Verification items for the finished model (mm, model axes). A direction names the side the tool comes from. Give positions to 0.01 mm unless a question says otherwise; leave off trailing zeros. Order: outer loops, then holes, each group sorted by start corner. A loop starts at its lowest first (then second) coordinate and runs counter-clockwise, first axis right, second up.
(1) Gauge pin test, flat ends, axial feed: pin 1 (12 mm diameter, centred on x = -10, z = 9.5, fed in from -Y); pin 2 (1.5 mm diameter, centred on x = 5, z = -1, fed in from -Y); pin 3 (5 mm diameter, centred on x = -10, z = -4, fed in from +Y); pin 4 (1.5 mm diameter, centred on y = 16, z = 3, fed in from +X). Record the tip position at first contact, or that the pin passes through.
(2) Access from +Z, -Z, +X, -X, +Y, -Y to the whole of each face (thin tool, end or side, straight path). Record for faces 1 (the face through (16, 0, 7)), 2 (the face through (-3, 25, 0)), 3 (the face through (0.867, 4.93, 3.905)).
(3) Scan lines: L1, parallel to Z at x = 0, y = 6.25; L2, parallel to X at y = 24.75, z = 0. Record each from-to range of solid material in increasing order.
(4) Sectioned sample at A-A on y = 5. Record the cut outline in (x, z), plus the area to 3 significant figures.
(5) Sectioned sample at D-D on y = 25. Record the cut outline in (x, z), plus the area to 3 significant figures.
(6) Sectioned sample at C-C on x = 0. Record the cut outline in (y, z).
(7) Sectioned sample at B-B on z = 0. Record the cut outline in (x, y).
Autodesk Inventor part; units mm, degrees
ref_plane "YZ Plane" through (0, 0, 0) normal (1, 0, 0) x (0, 1, 0)
ref_plane "XZ Plane" through (0, 0, 0) normal (0, 1, 0) x (-1, 0, 0)
ref_plane "XY Plane" through (0, 0, 0) normal (0, 0, 1) x (1, 0, 0)
sketch "Sketch1" plane through (0, 0, 0) normal (0, 1, 0) x (-1, 0, 0)
  circle A0 centre (0, 0) radius 4
  dimension "d0" = 8
extrude "Extrusion1" add sketch "Sketch1" along normal blind 12
sketch "Sketch2" plane through (0, 12, 0) normal (0, 1, 0) x (1, 0, 0)
  circle A0 centre (0, 0) radius 17
  circle A1 centre (0, 0) radius 4
  circle A2 centre (0, 0) radius 18
  dimension "d3" = 34
  dimension "d4" = 36
extrude "Extrusion2" add sketch "Sketch2" against normal blind 12 contours A2
sketch "Sketch4" plane through (0, 12, 0) normal (0, 1, 0) x (1, 0, 0)
  circle A0 centre (0, 0) radius 18
extrude "Extrusion3" add sketch "Sketch4" against normal blind 2
sketch "Sketch7" plane through (0, 12, 0) normal (0, 1, 0) x (1, 0, 0)
  circle A0 centre (0, 0) radius 5
  circle A1 centre (0, 0) radius 3
  dimension "d15" = 10
  dimension "d16" = 6
extrude "Extrusion6" add sketch "Sketch7" along normal blind 27
properties part number "kumandadış"
Ans:
1. pin 1: stops at y = 0
1. pin 2: stops at y = 10
1. pin 3: stops at y = 12
1. pin 4: stops at x = 4.47
2. face 1: +Z, -Z, +X, -X, -Y
2. face 2: +Y
2. face 3: -Y
3. L1: z = -18 to -17, -4 to 4, 17 to 18
3. L2: x = -5 to -3, 3 to 5
4. outline: circle Ø36 at (0, 0); circle Ø8 at (0, 0); hole circle Ø34 at (0, 0)
4. area: 160 mm2
5. outline: circle Ø10 at (0, 0); hole circle Ø6 at (0, 0)
5. area: 50.3 mm2
6. outline: (0, -18) - (12, -18) - (12, -5) - (39, -5) - (39, -3) - (12, -3) - (12, 3) - (39, 3) - (39, 5) - (12, 5) - (12, 18) - (0, 18) - (0, 17) - (10, 17) - (10, 4) - (0, 4) - (0, -4) - (10, -4) - (10, -17) - (0, -17) - close
7. outline: (-18, 0) - (-17, 0) - (-17, 10) - (-4, 10) - (-4, 0) - (4, 0) - (4, 10) - (17, 10) - (17, 0) - (18, 0) - (18, 12) - (5, 12) - (5, 39) - (3, 39) - (3, 12) - (-3, 12) - (-3, 39) - (-5, 39) - (-5, 12) - (-18, 12) - close
